Can you work these out from the model? Positions are in its coordinate system, mm. Give positions to 0.01 mm unless a question says otherwise; leave off trailing zeros. Loops run counter-clockwise (first coordinate to the right, second up) from the corner with the lowest first, then second, coordinate; pieces in that order, holes last. Notation, with made-up numbers: M -8,-5 L 51,-5 A14 cw 51,20 Z; hole C 1,-28.75 d10. An arc over 180 degrees is marked long. One line per item, written item: value. Start each with the question number.
Autodesk Inventor part; units mm, degrees
ref_plane "YZ Plane" through (0, 0, 0) normal (1, 0, 0) x (0, 1, 0)
ref_plane "XZ Plane" through (0, 0, 0) normal (0, 1, 0) x (-1, 0, 0)
ref_plane "XY Plane" through (0, 0, 0) normal (0, 0, 1) x (1, 0, 0)
sketch "Sketch2" plane through (0, 0, 0) normal (0, 0, 1) x (1, 0, 0)
  circle A0 centre (-4.95, 3) radius 1.5
  line L0 (0, 0) -> (-9.9, 0)
  line L1 (-9.9, 0) -> (-9.9, 300)
  line L2 (-9.9, 300) -> (0, 300)
  line L3 (0, 300) -> (0, 0)
  circle A1 centre (-4.95, 297) radius 1.5
  dimension "d53" = 3
  dimension "d54" = 9.9
  dimension "d55" = 300
  dimension "d56" = 3
extrude "Extrusion7" add sketch "Sketch2" along normal blind 5
properties part number "Cube_Holder_SB_V1_(71mm)"
Q1. If we section it at A-A, the plane x = -4.95: Write out the boundary of the cut face in (y, z), plus the area to 3 significant figures.
Q2. For P1, Ø1.8, axis at x = -4.95, y = 297, coming from the +Z side, with a flat end and sliding along its axis, tell me the tip position at first contact or that it passes through.
Q3. I need wall thicknesses on line 1 along Y through (x, z) = (-4.95, 3.6); line 2 along Y through (x, z) = (-6, 4); line 3 along X through (y, z) = (297, 2.1). Which ranges of each line are inside material? Lowest first, please.
Response:
1. outline: M 0,0 L 1.5,0 L 1.5,5 L 0,5 Z; M 4.5,0 L 295.5,0 L 295.5,5 L 4.5,5 Z; M 298.5,0 L 300,0 L 300,5 L 298.5,5 Z
1. area: 1,470 mm^2
2. P1: through
3. line 1: 0 to 1.5, 4.5 to 295.5, 298.5 to 300
3. line 2: 0 to 1.93, 4.07 to 295.93, 298.07 to 300
3. line 3: -9.9 to -6.45, -3.45 to 0
